CAD build for the part. Positions are in the model's coordinates, mm. Face numbers are marked on the shaded views. Give positions to 0.01 mm unless a question says otherwise; leave off trailing zeros. Order: outer loops, then holes, each group sorted by start corner. A loop starts at its lowest first (then second) coordinate and runs counter-clockwise, first axis right, second up. Notation, with made-up numbers: (87, 49) -> (117, 49) arc R26 ccw to (117, 78) -> close; hole circle Ø4 at (30, 34). An arc over 180 degrees is marked (long way). Answer as CSV lines item,"result".
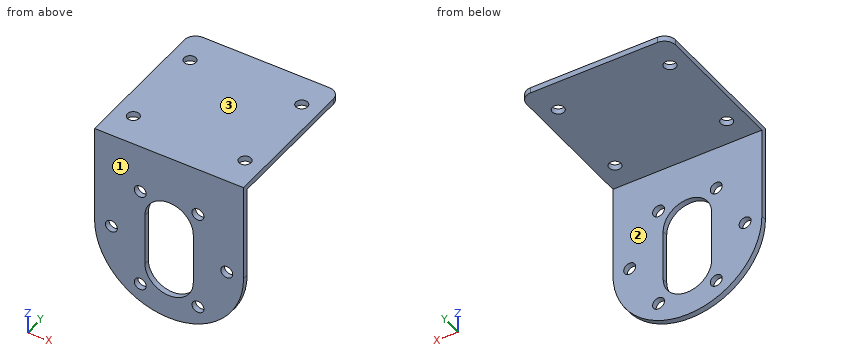
```python
from build123d import *

# Parameters (mm, degrees)
SKETCH_1_R          = 1.6
EXTRUDE_1_DEPTH     = 1.5
SKETCH_3_W          = 40
SKETCH_3_H          = 1.5
EXTRUDE_2_DEPTH     = 39.5
CUT_EXTRUDE_1_REACH = 67.14
SKETCH_4_R          = 1.6
FILLET_1_R          = 3


with BuildPart() as part:
    # 草图1 → 凸台-拉伸1 (new body)
    with BuildSketch(Plane(origin=(0, 0, 0), x_dir=(1, 0, 0), z_dir=(0, 1, 0))):
        with BuildLine():
            Line((-20, -13.25), (20, -13.25))
            Line((20, -13.25), (20, 13.25))
            ThreePointArc((20, 13.25), (0, 33.25), (-20, 13.25))
            Line((-20, 13.25), (-20, -13.25))
        make_face()
        with Locations(Location((15.5, 13.25, 0), (0, 0, 270))):
            Circle(SKETCH_1_R, mode=Mode.SUBTRACT)
        with Locations(Location((7.75, -0.173393759, 0), (0, 0, 270))):
            Circle(SKETCH_1_R, mode=Mode.SUBTRACT)
        with Locations(Location((-7.75, -0.173393759, 0), (0, 0, 270))):
            Circle(SKETCH_1_R, mode=Mode.SUBTRACT)
        with Locations(Location((-15.5, 13.25, 0), (0, 0, 270))):
            Circle(SKETCH_1_R, mode=Mode.SUBTRACT)
        with Locations(Location((-7.75, 26.673393759, 0), (0, 0, 270))):
            Circle(SKETCH_1_R, mode=Mode.SUBTRACT)
        with Locations(Location((7.75, 26.673393759, 0), (0, 0, 270))):
            Circle(SKETCH_1_R, mode=Mode.SUBTRACT)
        with BuildLine():
            Line((-6.5, 20.25), (-6.5, 6.25))
            ThreePointArc((-6.5, 6.25), (0, -0.25), (6.5, 6.25))
            Line((6.5, 6.25), (6.5, 20.25))
            ThreePointArc((6.5, 20.25), (0, 26.75), (-6.5, 20.25))
        make_face(mode=Mode.SUBTRACT)
    extrude(amount=EXTRUDE_1_DEPTH)

    # 草图3 → 凸台-拉伸2 (add)
    with BuildSketch(Plane(origin=(0, 1.5, 0), x_dir=(1, 0, 0), z_dir=(0, 1, 0))):
        with Locations((0, -12.5)):
            Rectangle(SKETCH_3_W, SKETCH_3_H)
    extrude(amount=EXTRUDE_2_DEPTH)

    # 草图4 → 切除-拉伸1 (cut, up to next)
    with BuildSketch(Plane.XY.offset(13.25), mode=Mode.PRIVATE) as cut_extrude_1_sk1:
        with Locations((-15, 32.5)):
            Circle(SKETCH_4_R)
    cut_extrude_1_tool1 = extrude(cut_extrude_1_sk1.sketch, amount=-CUT_EXTRUDE_1_REACH, mode=Mode.PRIVATE) & part.part
    # 草图4 → 切除-拉伸1 (cut, up to next)
    with BuildSketch(Plane.XY.offset(13.25), mode=Mode.PRIVATE) as cut_extrude_1_sk2:
        with Locations((15, 32.5)):
            Circle(SKETCH_4_R)
    cut_extrude_1_tool2 = extrude(cut_extrude_1_sk2.sketch, amount=-CUT_EXTRUDE_1_REACH, mode=Mode.PRIVATE) & part.part
    # 草图4 → 切除-拉伸1 (cut, up to next)
    with BuildSketch(Plane.XY.offset(13.25), mode=Mode.PRIVATE) as cut_extrude_1_sk3:
        with Locations((15, 8.5)):
            Circle(SKETCH_4_R)
    cut_extrude_1_tool3 = extrude(cut_extrude_1_sk3.sketch, amount=-CUT_EXTRUDE_1_REACH, mode=Mode.PRIVATE) & part.part
    # 草图4 → 切除-拉伸1 (cut, up to next)
    with BuildSketch(Plane.XY.offset(13.25), mode=Mode.PRIVATE) as cut_extrude_1_sk4:
        with Locations((-15, 8.5)):
            Circle(SKETCH_4_R)
    cut_extrude_1_tool4 = extrude(cut_extrude_1_sk4.sketch, amount=-CUT_EXTRUDE_1_REACH, mode=Mode.PRIVATE) & part.part
    add(cut_extrude_1_tool1.solids().sort_by_distance((-15, 32.5, 13.25))[0], mode=Mode.SUBTRACT)
    add(cut_extrude_1_tool2.solids().sort_by_distance((15, 32.5, 13.25))[0], mode=Mode.SUBTRACT)
    add(cut_extrude_1_tool3.solids().sort_by_distance((15, 8.5, 13.25))[0], mode=Mode.SUBTRACT)
    add(cut_extrude_1_tool4.solids().sort_by_distance((-15, 8.5, 13.25))[0], mode=Mode.SUBTRACT)

    # 圆角1
    fillet_1_edges = [part.edges().sort_by_distance(p)[0] for p in [
        (-20, 41, 12.5),
        (20, 41, 12.5),
    ]]
    fillet(fillet_1_edges, radius=FILLET_1_R)


solid = part.part
```
1) Pin check, flat tips, straight feed: P1, Ø10, axis at y = 7, z = -23.5, coming from the -X side; P2, Ø3, axis at x = -13, y = 21, coming from the -Z side; P3, Ø10, axis at x = 1.5, y = 5, coming from the -Z side; P4, Ø0.8, axis at y = 0.5, z = -15.5, coming from the -X side. Stop position of each tip, or through.
Data:
P1,"passes through"
P2,"stops at z = 11.75"
P3,"stops at z = -33.25"
P4,"stops at x = -19.91"
2) Pull direction Y, two halves, no side cores. Call the marked faces 1, 2 and 3: pulls with the +Y half, pulls with the -Y half, needs draft (parallel to the pull), parting line crosses it, or undercut.
Data:
face 1,"pulls with the -Y half"
face 2,"pulls with the +Y half"
face 3,"needs draft"
3) Band-saw the part on D-D, the plane x = -7.75. Write the cut outline in (y, z).
Data:
outline,"(0, -31.69) -> (1.5, -31.69) -> (1.5, -28.27) -> (0, -28.27) -> close; (0, -25.07) -> (1.5, -25.07) -> (1.5, -1.43) -> (0, -1.43) -> close; (0, 1.77) -> (1.5, 1.77) -> (1.5, 11.75) -> (41, 11.75) -> (41, 13.25) -> (0, 13.25) -> close"
4) Band-saw the part on B-B, the plane y = 32.5. Write the cut outline in (x, z).
Data:
outline,"(-20, 11.75) -> (-16.6, 11.75) -> (-16.6, 13.25) -> (-20, 13.25) -> close; (-13.4, 11.75) -> (13.4, 11.75) -> (13.4, 13.25) -> (-13.4, 13.25) -> close; (16.6, 11.75) -> (20, 11.75) -> (20, 13.25) -> (16.6, 13.25) -> close"
5) Band-saw the part on C-C, the plane x = 0. Write the cut outline in (y, z).
Data:
outline,"(0, -33.25) -> (1.5, -33.25) -> (1.5, -26.75) -> (0, -26.75) -> close; (0, 0.25) -> (1.5, 0.25) -> (1.5, 11.75) -> (41, 11.75) -> (41, 13.25) -> (0, 13.25) -> close"
6) Wall check: line 1 along Y through (x, z) = (18, -15.5); line 2 along Z through (x, y) = (-10, 11.5). Give the ranges that are in metal, low to high. Write a range as [from, to].
Data:
line 1,"y = [0, 1.5]"
line 2,"z = [11.75, 13.25]"
7) Band-saw the part on A-A, the plane z = -9. Write the cut outline in (x, y), then the cut area to 3 significant figures.
Data:
outline,"(-20, 0) -> (-6.5, 0) -> (-6.5, 1.5) -> (-20, 1.5) -> close; (6.5, 0) -> (20, 0) -> (20, 1.5) -> (6.5, 1.5) -> close"
area,"40.5 mm2"
